Check sheet for the modelled part. Datum: model origin and axes. Units: mm. A direction names the side the tool comes from. Coordinates: 2 decimals unless noted, no trailing zeros. Write each loop counter-clockwise with the first axis right and the second up, starting at its lowest first coordinate (ties: lowest second). Pieces come first, ordered by that corner, then holes. Notation, with made-up numbers: (-33.75, 65.5) - (-21.75, 65.5) arc R8 cw to (-21.75, 79.5) - close; hole circle Ø5 at (-26, 60). An arc over 180 degrees is marked (long way). Write each question's results on one line, items separated by ' | '.
from build123d import *

# Parameters (mm, degrees)
F1_DEPTH = 10


# Not quite as in the source:
# - a feature names something its author has since deleted; it is built from what else it names


with BuildPart() as f1:
    # F0 (on Top) → F1 (new body)
    with BuildSketch(Plane.XY):
        with BuildLine():
            ThreePointArc((-3.75, 0), (-3.3541019662, 1.6770509831), (-2.25, 3))
            Line((-2.25, 3), (-2.25, 11.6770509831))
            Line((-2.25, 11.6770509831), (-3.75, 11.6770509831))
            Line((-3.75, 11.6770509831), (-3.75, 0))
        make_face()
        with BuildLine():
            ThreePointArc((1.5, 1.6770509831), (2.0539595906, 0.9185586535), (2.25, 0))
            ThreePointArc((2.25, 0), (1.8708286934, -1.25), (0.8611111111, -2.0786985482))
            ThreePointArc((0.8611111111, -2.0786985482), (-1.25, -1.8708286934), (-2.25, 0))
            Line((-2.25, 0), (-2.25, 3))
            ThreePointArc((-2.25, 3), (-3.3541019662, 1.6770509831), (-3.75, 0))
            ThreePointArc((-3.75, 0), (0, -3.75), (3.75, 0))
            ThreePointArc((3.75, 0), (3.5575623677, 1.1858541226), (3, 2.25))
            ThreePointArc((3, 2.25), (2.3269511721, 2.9407139002), (1.5, 3.4369317712))
            Line((1.5, 3.4369317712), (1.5, 1.6770509831))
        make_face()
        with BuildLine():
            Line((1.5, 11.6770509831), (1.5, 3.4369317712))
            ThreePointArc((1.5, 3.4369317712), (2.3269511721, 2.9407139002), (3, 2.25))
            Line((3, 2.25), (3, 11.6770509831))
            Line((3, 11.6770509831), (1.5, 11.6770509831))
        make_face()
        with BuildLine():
            ThreePointArc((-2.25, 0), (-1.25, -1.8708286934), (0.8611111111, -2.0786985482))
            Line((0.8611111111, -2.0786985482), (-2.25, 0))
        make_face()
    extrude(amount=F1_DEPTH)


solid = f1.part
1. Access from +Z, -Z, +X, -X, +Y, -Y to the whole of each face (thin tool, end or side, straight path). Record for faces 1 (the flat face through (-2.25, 6, 5)), 2 (the flat face through (2, 11.677, 5)).
Values follow:
face 1: +Z, -Z, +Y | face 2: +Z, -Z, +X, -X, +Y
2. Sectioned sample at B-B (z = 8.75). Record the cut outline in (x, y).
Values follow:
outline: (-3.75, 0) arc R3.75 ccw (long way) to (3, 2.25) - (3, 11.68) - (1.5, 11.68) - (1.5, 1.68) arc R2.25 cw to (0.86, -2.08) - (-2.25, 0) - (-2.25, 11.68) - (-3.75, 11.68) - close
3. Sectioned sample at D-D (x = -1.25). Record the cut outline in (y, z), then the cut area to 3 significant figures.
Values follow:
outline: (-3.54, 0) - (-0.67, 0) - (-0.67, 10) - (-3.54, 10) - close | area: 28.7 mm^2
4. Go/stop test with flat-tipped pins: pin 1 (3 mm diameter, centred on y = 5, z = 6.5, fed in from +X); pin 2 (1 mm diameter, centred on x = -2, y = 0.5, fed in from +Z); pin 3 (1.5 mm diameter, centred on x = 0, z = 3.5, fed in from +Y). Record where each tip stops, or that it passes through.
Values follow:
pin 1: stops at x = 3 | pin 2: stops at z = 10 | pin 3: stops at y = -1
5. Material ranges on L1, parallel to X at y = 4.75, z = 7; L2, parallel to X at y = -3, z = 6; L3, parallel to X at y = -2, z = 7.25, recorded low to high. Write a range as [from, to].
Values follow:
L1: x = [-3.75, -2.25], [1.5, 3] | L2: x = [-2.25, 2.25] | L3: x = [-3.17, 0.74], [1.03, 3.17]
6. Sectioned sample at A-A (y = 2.75). Record the cut outline in (x, z), then the cut area to 3 significant figures.
Values follow:
outline: (-3.75, 0) - (-2.25, 0) - (-2.25, 10) - (-3.75, 10) - close; (1.5, 0) - (3, 0) - (3, 10) - (1.5, 10) - close | area: 30.0 mm^2
7. Draft check along X on faces 3 (the flat face through (-3.75, 6, 5)), 4 (the flat face through (-3, 11.677, 5)), 5 (the flat face through (3, 7, 5)), 6 (the flat face through (1.5, 7, 5)). Enter one of: pulls with the +X half, pulls with the -X half, needs draft (parallel to the pull), parting line crosses it, or undercut.
Values follow:
face 3: pulls with the -X half | face 4: needs draft | face 5: pulls with the +X half | face 6: undercut
8. Sectioned sample at C-C (y = -0.25). Record the cut outline in (x, z), then the cut area to 3 significant figures.
Values follow:
outline: (-3.74, 0) - (-1.88, 0) - (-1.88, 10) - (-3.74, 10) - close; (2.24, 0) - (3.74, 0) - (3.74, 10) - (2.24, 10) - close | area: 33.7 mm^2
